Check sheet for the modelled part. Datum: model origin and axes. Units: mm. Give positions to 0.01 mm unless a question says otherwise; leave off trailing zeros. Write each loop counter-clockwise with the first axis right and the second up, starting at its lowest first coordinate (ties: lowest second). Pieces come first, ordered by that corner, then holes. Notation, with made-up numbers: (-23.75, 27.5) -> (8.25, 27.5) arc R13 ccw to (8.25, 38.5) -> close; hole circle Ø9 at (-3.5, 33). An arc over 180 degrees is marked (long way). Answer as a JSON object with one key per item and string values.
from build123d import *

# Parameters (mm, degrees)
F1_DEPTH = 76.2


with BuildPart() as f1:
    # F0 (on Right) → F1 (new body)
    with BuildSketch(Plane.YZ):
        with BuildLine():
            ThreePointArc((64.744801, 0), (63.108078, 4.846023), (58.868258, 7.70727))
            ThreePointArc((58.868258, 7.70727), (48.759932, 0), (58.868258, -7.70727))
            ThreePointArc((58.868258, -7.70727), (63.108078, -4.846023), (64.744801, 0))
        make_face()
        with BuildLine():
            ThreePointArc((6.093416, -22.195651), (18.303388, -13.955738), (23.016877, 0))
            ThreePointArc((23.016877, 0), (18.303388, 13.955738), (6.093416, 22.195651))
            ThreePointArc((6.093416, 22.195651), (-23.016877, 0), (6.093416, -22.195651))
        make_face()
        with BuildLine():
            ThreePointArc((6.093416, 22.195651), (18.303388, 13.955738), (23.016877, 0))
            ThreePointArc((23.016877, 0), (18.303388, -13.955738), (6.093416, -22.195651))
            Line((6.093416, -22.195651), (58.868258, -7.70727))
            ThreePointArc((58.868258, -7.70727), (48.759932, 0), (58.868258, 7.70727))
            Line((58.868258, 7.70727), (6.093416, 22.195651))
        make_face()
    extrude(amount=F1_DEPTH)


solid = f1.part
1. Sectioned sample at C-C, the plane z = 10. Enter the section's corners in (x, y).
Determined:
{"outline": "(0, -20.73) -> (76.2, -20.73) -> (76.2, 50.52) -> (0, 50.52) -> close"}
2. Scan lines: L1, parallel to Z at x = 42, y = -3; L2, parallel to Z at x = 61, y = -15; L3, parallel to Y at x = 30, z = -6. Record each from-to range of solid material in increasing order. Write a range as [from, to].
Determined:
{"L1": "[-22.82, 22.82]", "L2": "[-17.46, 17.46]", "L3": "[-22.22, 62.03]"}
3. Sectioned sample at B-B, the plane y = 41.5. Enter the section's corners in (x, z), plus the area to 3 significant figures.
Determined:
{"outline": "(0, -12.48) -> (76.2, -12.48) -> (76.2, 12.48) -> (0, 12.48) -> close", "area": "1,900 mm^2"}
4. Go/stop test with flat-tipped pins: P1, Ø4, axis at x = 36, z = 17.5, coming from the -Y side; P2, Ø2, axis at x = 28, z = 13.5, coming from the -Y side; P3, Ø2, axis at x = 39, y = 35, coming from the -Z side. Record where each tip stops, or that it passes through.
Determined:
{"P1": "y = -17.02", "P2": "y = -19.33", "P3": "z = -14.53"}
5. Sectioned sample at A-A, the plane x = 44. Enter the section's corners in (y, z), plus the area to 3 significant figures.
Determined:
{"outline": "(6.09, -22.2) -> (58.87, -7.71) arc R7.99 ccw to (58.87, 7.71) -> (6.09, 22.2) arc R23.02 ccw (long way) to start", "area": "2,750 mm^2"}
